```python
from build123d import *

# Parameters (mm, degrees)
SK_PLATE_W           = 56
SK_PLATE_H           = 56
EX_PLATE_DEPTH       = 3
SK_STANDOFFS_R       = 3
EX_STANDOFFS_DEPTH   = 5
SK_INSERTS_M3_R      = 2
CUT_INSERTS_M3_DEPTH = 5.7
SK_PANHOLES_R        = 2.15
CUT_PANHOLES_DEPTH   = 3


with BuildPart() as part:
    # SK_Plate → EX_Plate (new body)
    with BuildSketch(Plane(origin=(0, 0, 0), x_dir=(1, 0, 0), z_dir=(0, 1, 0))):
        Rectangle(SK_PLATE_W, SK_PLATE_H)
    extrude(amount=EX_PLATE_DEPTH)

    # SK_Standoffs → EX_Standoffs (add)
    with BuildSketch(Plane(origin=(0, 3, 0), x_dir=(1, 0, 0), z_dir=(0, 1, 0))):
        with Locations(Location((22.5, -22.5, 0), (0, 0, 270))):
            Circle(SK_STANDOFFS_R)
        with Locations(Location((-22.5, -22.5, 0), (0, 0, 270))):
            Circle(SK_STANDOFFS_R)
        with Locations(Location((22.5, 22.5, 0), (0, 0, 270))):
            Circle(SK_STANDOFFS_R)
        with Locations(Location((-22.5, 22.5, 0), (0, 0, 270))):
            Circle(SK_STANDOFFS_R)
    extrude(amount=EX_STANDOFFS_DEPTH)

    # SK_Inserts_M3 → CUT_Inserts_M3 (cut)
    with BuildSketch(Plane(origin=(0, 8, 0), x_dir=(1, 0, 0), z_dir=(0, 1, 0))):
        with Locations(Location((22.5, -22.5, 0), (0, 0, 270))):
            Circle(SK_INSERTS_M3_R)
        with Locations(Location((-22.5, -22.5, 0), (0, 0, 270))):
            Circle(SK_INSERTS_M3_R)
        with Locations(Location((22.5, 22.5, 0), (0, 0, 270))):
            Circle(SK_INSERTS_M3_R)
        with Locations(Location((-22.5, 22.5, 0), (0, 0, 270))):
            Circle(SK_INSERTS_M3_R)
    extrude(amount=-CUT_INSERTS_M3_DEPTH, mode=Mode.SUBTRACT)

    # SK_PanHoles → CUT_PanHoles (cut)
    with BuildSketch(Plane(origin=(0, 0, 0), x_dir=(1, 0, 0), z_dir=(0, 1, 0))):
        with Locations(Location((0, -24, 0), (0, 0, 270))):
            Circle(SK_PANHOLES_R)
        with Locations(Location((0, 24, 0), (0, 0, 270))):
            Circle(SK_PANHOLES_R)
    extrude(amount=CUT_PANHOLES_DEPTH, mode=Mode.SUBTRACT)


solid = part.part
```
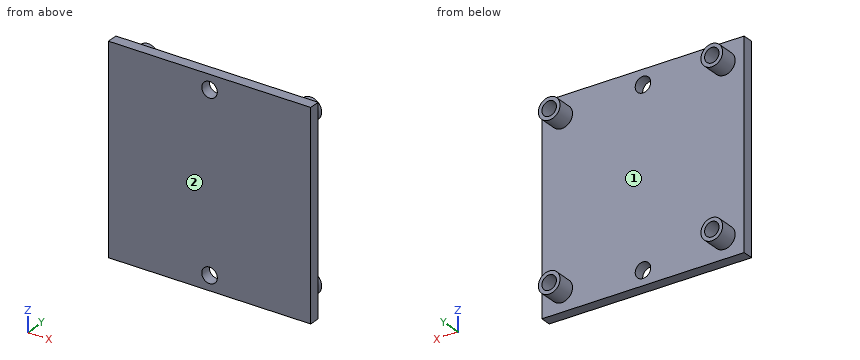
Read the model definition and answer for the solid it produces. Units are mm, in the model's axes. Face numbers are marked on the shaded views. A direction names the side the tool comes from. Coordinates: 2 decimals unless noted, no trailing zeros. Write each loop counter-clockwise with the first axis right and the second up, starting at its lowest first coordinate (ties: lowest second). Pieces come first, ordered by that corner, then holes. Notation, with made-up numbers: (-9, 87.25) -> (-5, 87.25) arc R30 ccw to (-5, 114.25) -> close; hole circle Ø9 at (50, -39.5). An arc over 180 degrees is marked (long way). Return JSON: item names as keys, results as strings.
1. A cutting plane is placed at B-B (z = -22.5). Determine the outline of the cut face in (x, y), and give its area (3 significant figures).
Found:
{"outline": "(-28, 0) -> (-1.54, 0) -> (-1.54, 3) -> (-19.5, 3) -> (-19.5, 8) -> (-20.5, 8) -> (-20.5, 2.3) -> (-24.5, 2.3) -> (-24.5, 8) -> (-25.5, 8) -> (-25.5, 3) -> (-28, 3) -> close; (1.54, 0) -> (28, 0) -> (28, 3) -> (25.5, 3) -> (25.5, 8) -> (24.5, 8) -> (24.5, 2.3) -> (20.5, 2.3) -> (20.5, 8) -> (19.5, 8) -> (19.5, 3) -> (1.54, 3) -> close", "area": "173 mm2"}
2. A cutting plane is placed at C-C (x = 22.5). Determine the outline of the cut face in (y, z).
Found:
{"outline": "(0, -28) -> (3, -28) -> (3, -25.5) -> (8, -25.5) -> (8, -24.5) -> (2.3, -24.5) -> (2.3, -20.5) -> (8, -20.5) -> (8, -19.5) -> (3, -19.5) -> (3, 19.5) -> (8, 19.5) -> (8, 20.5) -> (2.3, 20.5) -> (2.3, 24.5) -> (8, 24.5) -> (8, 25.5) -> (3, 25.5) -> (3, 28) -> (0, 28) -> close"}
3. Each of these flat-tipped pins is pushed along its axis until it touches: P1, Ø3.5, axis at x = 0, z = 24, coming from the +Y side; P2, Ø6.5, axis at x = -22.5, z = -22.5, coming from the -Y side; P3, Ø8, axis at x = -3, z = 1, coming from the +Y side; P4, Ø2, axis at x = 23, z = 22, coming from the +Y side. Where does it stop, or does it pass through?
Found:
{"P1": "through", "P2": "y = 0", "P3": "y = 3", "P4": "y = 2.3"}
4. A tool of negligible diameter and unlimited length cuts with its end or side. For the marked faces 1 and 2, from which of +Z, -Z, +X, -X, +Y, -Y can it reach the whole face along a straight path? Write none if from no direction.
Found:
{"face 1": "+Y", "face 2": "+Z, -Z, +X, -X, -Y"}
5. A cutting plane is placed at A-A (y = 6). Determine the outline of the cut face in (x, z).
Found:
{"outline": "circle Ø6 at (-22.5, -22.5); circle Ø6 at (-22.5, 22.5); circle Ø6 at (22.5, -22.5); circle Ø6 at (22.5, 22.5); hole circle Ø4 at (-22.5, -22.5); hole circle Ø4 at (-22.5, 22.5); hole circle Ø4 at (22.5, -22.5); hole circle Ø4 at (22.5, 22.5)"}
6. A cutting plane is placed at D-D (z = 1.5). Determine the outline of the cut face in (x, y).
Found:
{"outline": "(-28, 0) -> (28, 0) -> (28, 3) -> (-28, 3) -> close"}
7. Find the intervals of material crossed by line 1 along X through (y, z) = (3.5, 22.5); line 2 along Z through (x, y) = (24, 3.75); line 3 along Y through (x, z) = (24.5, 9.5), in increasing order. Write a range as from..to.
Found:
{"line 1": "-25.5..-24.5, -20.5..-19.5, 19.5..20.5, 24.5..25.5", "line 2": "-25.1..-23.82, -21.18..-19.9, 19.9..21.18, 23.82..25.1", "line 3": "0..3"}
